Check sheet for the modelled part. Datum: model origin and axes. Units: mm. A direction names the side the tool comes from. Coordinates: 2 decimals unless noted, no trailing zeros. Loops run counter-clockwise (first coordinate to the right, second up) from the corner with the lowest first, then second, coordinate; pieces in that order, holes last.
Autodesk Inventor part; units mm, degrees
ref_plane "YZ Plane" through (0, 0, 0) normal (1, 0, 0) x (0, 1, 0)
ref_plane "XZ Plane" through (0, 0, 0) normal (0, 1, 0) x (-1, 0, 0)
ref_plane "XY Plane" through (0, 0, 0) normal (0, 0, 1) x (1, 0, 0)
sketch "스케치1" plane through (0, 0, 0) normal (0, 0, 1) x (1, 0, 0)
  circle A0 centre (0, 0) radius 1.5
  circle A1 centre (0, 0) radius 2.9
  dimension "d0" = 3
  dimension "d1" = 5.8
extrude "돌출1" add sketch "스케치1" along normal blind 1.5
sketch "스케치2" plane through (0, 0, 0) normal (0, 0, -1) x (-1, 0, 0)
  line L0 (7.6095, 2.163) -> (0.8412, 12.6915)
  line L1 (-0.8412, 12.6915) -> (-7.6095, 2.163)
  line L2 (7.6095, -2.163) -> (0.8412, -12.6915)
  line L3 (-0.8412, -12.6915) -> (-7.6095, -2.163)
  circle A0 centre (0, 10.1) radius 1.1
  circle A1 centre (0, -10.1) radius 1.1
  arc A2 (0.8412, 12.6915) -> (-0.8412, 12.6915) centre (0, 12.1507) ccw
  arc A3 (-0.8412, -12.6915) -> (0.8412, -12.6915) centre (0, -12.1507) ccw
  arc A4 (7.6095, -2.163) -> (7.6095, 2.163) centre (4.2448, 0) ccw
  arc A5 (-7.6095, 2.163) -> (-7.6095, -2.163) centre (-4.2448, 0) ccw
  circle A6 centre (0, 0) radius 1.5
  dimension "d8" = 2.2
  dimension "d9" = 2.2
  dimension "d10" = 10.1
  dimension "d11" = 10.1
  dimension "d12" = 1
  dimension "d13" = 4
extrude "돌출2" add sketch "스케치2" along normal blind 1.8
sketch "스케치3" plane through (0, 0, -1.8) normal (0, 0, -1) x (-1, 0, 0)
  circle A0 centre (0, 0) radius 1.5
  circle A1 centre (0, -10.1) radius 1.1
  circle A2 centre (0, 10.1) radius 1.1
  line L0 (-0.8412, 12.6915) -> (-7.6095, 2.163)
  arc A3 (-7.6095, 2.163) -> (-7.6095, -2.163) centre (-4.2448, 0) ccw
  line L1 (-7.6095, -2.163) -> (-0.8412, -12.6915)
  arc A4 (-0.8412, -12.6915) -> (0.8412, -12.6915) centre (0, -12.1507) ccw
  line L2 (0.8412, -12.6915) -> (7.6095, -2.163)
  arc A5 (7.6095, -2.163) -> (7.6095, 2.163) centre (4.2448, 0) ccw
  line L3 (7.6095, 2.163) -> (0.8412, 12.6915)
  arc A6 (0.8412, 12.6915) -> (-0.8412, 12.6915) centre (0, 12.1507) ccw
  circle A7 centre (0, 0) radius 1.5
  circle A8 centre (0, 0) radius 7.5
  dimension "d16" = 15
extrude "돌출3" add sketch "스케치3" along normal blind 10 contours A0 | A8
sketch "스케치4" plane through (0, 0, -11.8) normal (0, 0, -1) x (-1, 0, 0)
  circle A0 centre (0, 0) radius 7.5
  circle A1 centre (0, 0) radius 7.6
  dimension "d19" = 0.1
extrude "돌출4" add sketch "스케치4" along normal blind 9 contours A0 | A1
properties part number "GM15BY_StepMotor"
1) Set-up check for faces 1 (the cylindrical face through (8.245, -0.032, -0.887)), 2 (the cylindrical face through (7.493, -0.33, -6.73)), 3 (the flat face through (0, 0, -20.8)), 4 (the flat face through (0.1, 3.1, 0)), 5 (the cylindrical face through (7.593, -0.334, -16.237)): record each of +Z, -Z, +X, -X, +Y, -Y from which the full face is reachable in a straight line by a thin tool's end or side.
Answer sheet:
face 1: +Z, -Z, +X
face 2: none
face 3: -Z, +X, -X, +Y, -Y
face 4: +Z
face 5: -Z
2) Mould release check, pull along X, two halves, no side actions. Record for faces 6 (the cylindrical face through (-8.245, 0.032, -0.887)), 7 (the cylindrical face through (-0.508, 11.076, -0.887)), 8 (the cylindrical face through (-2.9, -0.1, 0.7)), 9 (the cylindrical face through (0, -9, -1)): +X half, -X half, draft (parallel to the pull), parting line (faces both ways), or undercut.
Answer sheet:
face 6: -X half
face 7: undercut
face 8: parting line
face 9: undercut
3) Depth check by flat-ended pin: pin 1 (1.8 mm diameter, centred on x = 0, y = -10.1, fed in from -Z); pin 2 (6 mm diameter, centred on x = -5, y = -5.5, fed in from +Z); pin 3 (1.5 mm diameter, centred on x = 0, y = -0.5, fed in from +Z); pin 4 (10 mm diameter, centred on y = 0.5, z = -10, fed in from -X). Enter the tip coordinate at first touch or a pass-through.
Answer sheet:
pin 1: passes through
pin 2: stops at z = 0
pin 3: stops at z = -1.8
pin 4: stops at x = -7.6
4) Scan lines: line 1 (Y direction, x = 0, z = -0.7); line 2 (Y direction, x = 0, z = 0.9); line 3 (Z direction, x = 0, y = -5). Record each from-to range of solid material in increasing order.
Answer sheet:
line 1: y = -13.15 to -11.2, -9 to -1.5, 1.5 to 9, 11.2 to 13.15
line 2: y = -2.9 to -1.5, 1.5 to 2.9
line 3: z = -20.8 to 0
5) Section check B-B on y = 10.1. Enter the section's corners in (x, z), plus the area to 3 significant figures.
Answer sheet:
outline: (-2.51, -1.8) - (-1.1, -1.8) - (-1.1, 0) - (-2.51, 0) - close; (1.1, -1.8) - (2.51, -1.8) - (2.51, 0) - (1.1, 0) - close
area: 5.07 mm2
6) Section check A-A on z = -1.25. Enter the section's corners in (x, y).
Answer sheet:
outline: (-7.61, -2.16) - (-0.84, -12.69) arc R1 ccw to (0.84, -12.69) - (7.61, -2.16) arc R4 ccw to (7.61, 2.16) - (0.84, 12.69) arc R1 ccw to (-0.84, 12.69) - (-7.61, 2.16) arc R4 ccw to start; hole circle Ø3 at (0, 0); hole circle Ø2.2 at (0, -10.1); hole circle Ø2.2 at (0, 10.1)
7) Section check C-C on y = 0. Enter the section's corners in (x, z).
Answer sheet:
outline: (-8.24, -1.8) - (-7.5, -1.8) - (-7.5, -11.8) - (-7.6, -11.8) - (-7.6, -20.8) - (7.6, -20.8) - (7.6, -11.8) - (7.5, -11.8) - (7.5, -1.8) - (8.24, -1.8) - (8.24, 0) - (2.9, 0) - (2.9, 1.5) - (1.5, 1.5) - (1.5, -1.8) - (-1.5, -1.8) - (-1.5, 1.5) - (-2.9, 1.5) - (-2.9, 0) - (-8.24, 0) - close
8) Section check D-D on z = -15. Enter the section's corners in (x, y), plus the area to 3 significant figures.
Answer sheet:
outline: circle Ø15.2 at (0, 0)
area: 181 mm2
